Geometry check sheet. Reference: drawing and pictorial views, mm from the part's lowest x, y, z. A direction names the side the tool comes from. Coordinates: 2 decimals unless noted, no trailing zeros. Loops run counter-clockwise (first coordinate to the right, second up) from the corner with the lowest first, then second, coordinate; pieces in that order, holes last.
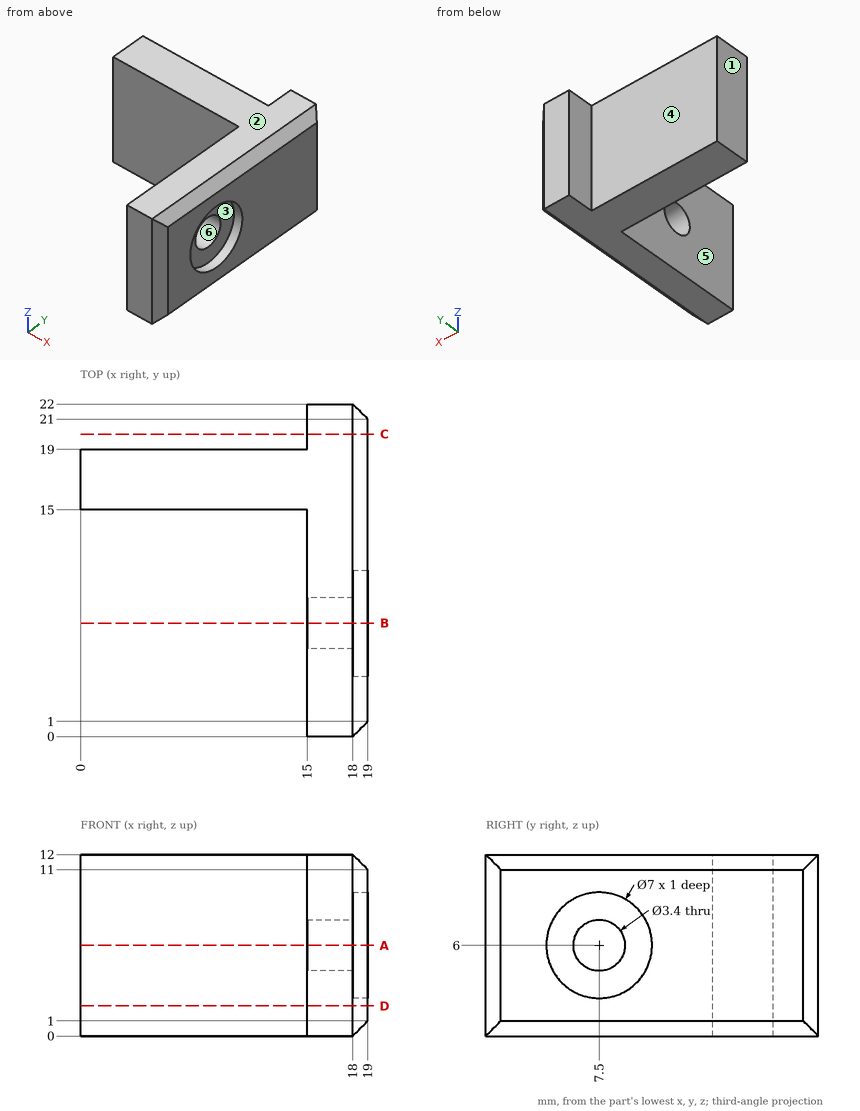
1) Section check A-A on z = 6. Record the cut outline in (x, y), and give its area (3 significant figures).
Data:
outline: (0, 15) - (15, 15) - (15, 9.2) - (18, 9.2) - (18, 11) - (19, 11) - (19, 21) - (18, 22) - (15, 22) - (15, 19) - (0, 19) - close; (15, 0) - (18, 0) - (19, 1) - (19, 4) - (18, 4) - (18, 5.8) - (15, 5.8) - close
area: 130 mm2
2) Section check B-B on y = 7.5. Record the cut outline in (x, z).
Data:
outline: (15, 0) - (18, 0) - (19, 1) - (19, 2.5) - (18, 2.5) - (18, 4.3) - (15, 4.3) - close; (15, 7.7) - (18, 7.7) - (18, 9.5) - (19, 9.5) - (19, 11) - (18, 12) - (15, 12) - close
3) Depth check by flat-ended pin: pin 1 (2 mm diameter, centred on x = 9, z = 6, fed in from +Y); pin 2 (6 mm diameter, centred on y = 7, z = 6, fed in from -X); pin 3 (4 mm diameter, centred on y = 7.5, z = 6, fed in from +X). Enter the tip coordinate at first touch or a pass-through.
Data:
pin 1: stops at y = 19
pin 2: stops at x = 15
pin 3: stops at x = 18
4) Material ranges on probe 1 along Y at (x, z) = (16.6, 6); probe 2 along Y at (x, z) = (6.25, 11.5), recorded low to high.
Data:
probe 1: y = 0 to 5.8, 9.2 to 22
probe 2: y = 15 to 19
5) Section check C-C on y = 20. Record the cut outline in (x, z), and give its area (3 significant figures).
Data:
outline: (15, 0) - (18, 0) - (19, 1) - (19, 11) - (18, 12) - (15, 12) - close
area: 47.0 mm2
6) Section check D-D on z = 2. Record the cut outline in (x, y).
Data:
outline: (0, 15) - (15, 15) - (15, 0) - (18, 0) - (19, 1) - (19, 21) - (18, 22) - (15, 22) - (15, 19) - (0, 19) - close
7) Access from +Z, -Z, +X, -X, +Y, -Y to the whole of each face (thin tool, end or side, straight path). Record for the marked faces 4, 5 and 6.
Data:
face 4: +Z, -Z, -X, +Y
face 5: +Z, -Z, -X, -Y
face 6: +X, -X
8) Mould release check, pull along Z, two halves, no side actions. Record for the marked faces 1, 2 and 3: +Z half, -Z half, draft (parallel to the pull), parting line (faces both ways), or undercut.
Data:
face 1: draft
face 2: +Z half
face 3: undercut
